from build123d import *

# Parameters (mm, degrees)
ESBO_O1_W                = 45
ESBO_O1_H                = 9
RESSALTO_EXTRUS_O2_DEPTH = 10
RESSALTO_EXTRUS_O3_DEPTH = 12
ESBO_O2_R                = 2
ESBO_O2_W                = 30
ESBO_O2_H                = 7
CORTE_EXTRUS_O4_DEPTH    = 9
FILETE2_R                = 2


with BuildPart() as part:
    # Esboço1 → Ressalto-extrusão2 (new body)
    with BuildSketch(Plane.XY):
        with Locations((32.5, 0)):
            Rectangle(ESBO_O1_W, ESBO_O1_H)
        with BuildLine():
            ThreePointArc((30, -1.5), (28.5, 0), (30, 1.5))
            Line((30, 1.5), (50, 1.5))
            ThreePointArc((50, 1.5), (51.5, 0), (50, -1.5))
            Line((50, -1.5), (30, -1.5))
        make_face(mode=Mode.SUBTRACT)
        Polygon((6, 4.5), (-6, 4.5), (-10, 4.5), (-10, -4.5), (10, -4.5), (10, 4.5), align=None)
        with Locations((-32.5, 0)):
            Rectangle(ESBO_O1_W, ESBO_O1_H)
        with BuildLine():
            ThreePointArc((-50, -1.5), (-51.5, 0), (-50, 1.5))
            Line((-50, 1.5), (-30, 1.5))
            ThreePointArc((-30, 1.5), (-28.5, 0), (-30, -1.5))
            Line((-30, -1.5), (-50, -1.5))
        make_face(mode=Mode.SUBTRACT)
    extrude(amount=RESSALTO_EXTRUS_O2_DEPTH)

    # Esboço1<5> → Ressalto-extrusão3 (add)
    with BuildSketch(Plane.XY):
        Polygon((6, 4.5), (-6, 4.5), (-10, 4.5), (-10, -4.5), (10, -4.5), (10, 4.5), align=None)
        Polygon((-10, 4.5), (-6, 4.5), (-6, 11.5), (6, 11.5), (6, 4.5), (10, 4.5), (10, 13.5), (-10, 13.5), align=None)
    extrude(amount=-RESSALTO_EXTRUS_O3_DEPTH)

    # Esboço2 → Corte-extrusão4 (cut)
    with BuildSketch(Plane(origin=(0, 4.5, 0), x_dir=(1, 0, 0), z_dir=(0, 1, 0))):
        with Locations((-19, -5)):
            Circle(ESBO_O2_R)
        with Locations((16, -5)):
            Circle(ESBO_O2_R)
        with Locations((40, -3.5)):
            Rectangle(ESBO_O2_W, ESBO_O2_H)
    extrude(amount=-CORTE_EXTRUS_O4_DEPTH, mode=Mode.SUBTRACT)

    # Filete2
    filete2_edges = [part.edges().sort_by_distance(p)[0] for p in [
        (-10, 0, 0),
        (10, 0, 0),
        (-10, 4.5, -12),
        (10, 4.5, -12),
        (25, 0, 0),
        (25, 0, 7),
    ]]
    fillet(filete2_edges, radius=FILETE2_R)


solid = part.part
Can you work these out from the model? Positions are in its coordinate system, mm. A direction names the side the tool comes from. Coordinates: 2 decimals unless noted, no trailing zeros. Order: outer loops, then holes, each group sorted by start corner. A loop starts at its lowest first (then second) coordinate and runs counter-clockwise, first axis right, second up. Notation, with made-up numbers: M 38.25,80 L 87.25,80 A15 cw 87.25,97 Z; hole C 43,38 d7. An arc over 180 degrees is marked long. Write item = value, one per line.
(1) Suppose I cut it at A-A on y = 0. Please give me the cut outline in (x, z).
Results are:
outline = M -55,0 L -51.5,0 L -51.5,10 L -55,10 Z; M -28.5,0 L -12,0 A2 cw -10,-2 L -10,-10 A2 ccw -8,-12 L 8,-12 A2 ccw 10,-10 L 10,-2 A2 cw 12,0 L 23,0 A2 ccw 25,2 L 25,5 A2 cw 27,7 L 28.5,7 L 28.5,10 L -28.5,10 Z; M 51.5,7 L 55,7 L 55,10 L 51.5,10 Z; hole C -19,5 d4; hole C 16,5 d4
(2) Suppose I cut it at B-B on x = 16. Please give me the cut outline in (y, z), plus the area to 3 significant figures.
Results are:
outline = M -4.5,0 L 4.5,0 L 4.5,3 L -4.5,3 Z; M -4.5,7 L 4.5,7 L 4.5,10 L -4.5,10 Z
area = 54.0 mm2
(3) If we mould it in two halves opening along Y, with no side actions, what happens to faces 4 (the face through (-13, -4.5, 4)), 5 (the face through (10.6, 0.06, -0.57)), 6 (the face through (-51.5, 0, 4.9)), 7 (the face through (40, 1.5, 8))? For each: pulls with the +Y half, pulls with the -Y half, needs draft (parallel to the pull), parting line crosses it, or undercut.
Results are:
face_4 = pulls with the -Y half
face_5 = needs draft
face_6 = undercut
face_7 = undercut
(4) Suppose I cut it at D-D on z = -7. Please give me the cut outline in (x, y).
Results are:
outline = M -10,-4.5 L 10,-4.5 L 10,13.5 L -10,13.5 Z; hole M -6,4.5 L 6,4.5 L 6,11.5 L -6,11.5 Z
(5) For faces 1 (the face through (41, 2, 7)), 2 (the face through (0, 12, 0)), 3 (the face through (51.5, 0, 8.5)), which set-ups out of +Z, -Z, +X, -X, +Y, -Y let a thin tool reach every point of the face, with its end or its side?
Results are:
face_1 = -Z, +X, +Y, -Y
face_2 = +Z, +X, -X, +Y
face_3 = +Z, -Z
(6) Suppose I cut it at C-C on y = 5.5. Please give me the cut outline in (x, z).
Results are:
outline = M -10,-10 A2 ccw -8,-12 L -6,-12 L -6,0 L -10,0 Z; M 6,-12 L 8,-12 A2 ccw 10,-10 L 10,0 L 6,0 Z
(7) For pin 1 Ø7 at (x, y) = (-36, -2) entering from -Z; pin 2 Ø2.5 at (x, z) = (39, 9) entering from +Y; pin 3 Ø5 at (y, z) = (2, -6.5) entering from -X, each with a flat end and sliding along its axis, tell me the tip position at first contact or that it passes through.
Results are:
pin_1 = 0
pin_2 = 4.5
pin_3 = -10
(8) I need wall thicknesses on line 1 along X through (y, z) = (1.75, 5.25); line 2 along X through (y, z) = (0, 5); line 3 along Y through (x, z) = (-5.5, -3.25). Which ranges of each line are inside material? Lowest first, please. Write a range as [from, to].
Results are:
line_1 = [-55, -20.98], [-17.02, 14.02], [17.98, 25.02]
line_2 = [-55, -51.5], [-28.5, -21], [-17, 14], [18, 25]
line_3 = [-4.5, 4.5], [11.5, 13.5]
